Check sheet for the modelled part. Datum: model origin and axes. Units: mm. Face numbers are marked on the shaded views. A direction names the side the tool comes from. Round coordinates to 2 decimals unless told otherwise and drop trailing zeros. Write each loop counter-clockwise with the first axis right and the second up, starting at its lowest first coordinate (ties: lowest second). Pieces come first, ordered by that corner, then holes. Notation, with made-up numbers: (82, 42) -> (114, 42) arc R10 ccw to (114, 50) -> close; hole circle Ø1 at (59, -35.5). An arc over 180 degrees is marked (long way). One line per item, written item: value.
from build123d import *

# Parameters (mm, degrees)
SKIZZE1_W                       = 9.5
SKIZZE1_H                       = 11.093
SKIZZE1_W_2                     = 8.7
SKIZZE1_H_2                     = 4.7
SKIZZE1_H_3                     = 5.193
AUFSATZ_LINEAR_AUSTRAGEN1_DEPTH = 19.7
AUFSATZ_LINEAR_AUSTRAGEN2_DEPTH = 2.3
SCHNITT_LINEAR_AUSTRAGEN1_DEPTH = 13.7
SKIZZE4_W                       = 13.3
SKIZZE4_H                       = 5.193
SCHNITT_LINEAR_AUSTRAGEN2_DEPTH = 0.4
AUFSATZ_LINEAR_AUSTRAGEN3_DEPTH = 14.1
AUFSATZ_LINEAR_START            = -9.5
AUFSATZ_LINEAR_AUSTRAGEN4_DEPTH = 9.5
SCHNITT_LINEAR_AUSTRAGEN3_REACH = 39.021
SKIZZE7_W                       = 8.7
SKIZZE7_H                       = 0.4
SKIZZE8_W                       = 10
SKIZZE8_H                       = 5
AUFSATZ_LINEAR_AUSTRAGEN5_DEPTH = 0.4


with BuildPart() as part:
    # Skizze1 → Aufsatz-Linear austragen1 (new body)
    with BuildSketch(Plane(origin=(0, 0, 0), x_dir=(1, 0, 0), z_dir=(0, 1, 0))):
        with Locations((4.75, 5.5465)):
            Rectangle(SKIZZE1_W, SKIZZE1_H)
        with Locations((4.75, 2.75)):
            Rectangle(SKIZZE1_W_2, SKIZZE1_H_2, mode=Mode.SUBTRACT)
        with Locations((4.75, 8.0965)):
            Rectangle(SKIZZE1_W_2, SKIZZE1_H_3, mode=Mode.SUBTRACT)
    extrude(amount=AUFSATZ_LINEAR_AUSTRAGEN1_DEPTH)

    # Skizze2 → Aufsatz-Linear austragen2 (add)
    with BuildSketch(Plane.ZY):
        Polygon((-11.093, 0), (-8.093, 10.13), (-5.093, 0), align=None)
    aufsatz_linear_austragen2 = extrude(amount=AUFSATZ_LINEAR_AUSTRAGEN2_DEPTH)

    # Spiegeln1: Aufsatz-Linear austragen2 across plane
    add(aufsatz_linear_austragen2.mirror(Plane(origin=(4.75, 0, 0), x_dir=(0, 0, 1), z_dir=(1, 0, 0))))

    # Skizze3 → Schnitt-Linear austragen1 (cut)
    with BuildSketch(Plane.ZY.offset(2.3)):
        Polygon((-10.379677593, 1), (-5.806322407, 1), (-8.093, 8.721348004), align=None)
    extrude(amount=-SCHNITT_LINEAR_AUSTRAGEN1_DEPTH, mode=Mode.SUBTRACT)

    # Skizze4 → Schnitt-Linear austragen2 (cut)
    with BuildSketch(Plane.XZ):
        with Locations((4.75, -8.0965)):
            Rectangle(SKIZZE4_W, SKIZZE4_H)
    extrude(amount=-SCHNITT_LINEAR_AUSTRAGEN2_DEPTH, mode=Mode.SUBTRACT)

    # Skizze5 → Aufsatz-Linear austragen3 (add)
    with BuildSketch(Plane.ZY.offset(2.3)):
        Polygon((-20.977529946, -17.120508076), (-20.631119785, -17.320508076), (-10.631119785, 0), (-11.093, 0), align=None)
    extrude(amount=-AUFSATZ_LINEAR_AUSTRAGEN3_DEPTH)

    # Skizze6 → Aufsatz-Linear austragen4 (add)
    with BuildSketch(Plane.ZY.offset(AUFSATZ_LINEAR_START)):
        Polygon((-20.977529946, -17.120508076), (-11.093, 0), (-11.093, 14.7), align=None)
    extrude(amount=AUFSATZ_LINEAR_AUSTRAGEN4_DEPTH)

    # Skizze7 → Schnitt-Linear austragen3 (cut, up to next)
    with BuildSketch(Plane(origin=(0, 19.7, 0), x_dir=(1, 0, 0), z_dir=(0, 1, 0)), mode=Mode.PRIVATE) as schnitt_linear_austragen3_sk1:
        with Locations((4.75, 5.3)):
            Rectangle(SKIZZE7_W, SKIZZE7_H)
    schnitt_linear_austragen3_tool1 = extrude(schnitt_linear_austragen3_sk1.sketch, amount=-SCHNITT_LINEAR_AUSTRAGEN3_REACH, mode=Mode.PRIVATE) & part.part
    add(schnitt_linear_austragen3_tool1.solids().sort_by_distance((4.75, 19.7, -5.3))[0], mode=Mode.SUBTRACT)

    # Skizze8 → Aufsatz-Linear austragen5 (add)
    with BuildSketch(Plane(origin=(0, 4.603409902, -7.973339838), x_dir=(1, 0, 0), z_dir=(0, -0.5, 0.866025404))):
        with Locations((-7.3, -22.815559892)):
            Rectangle(SKIZZE8_W, SKIZZE8_H)
        with Locations((16.8, -22.815559892)):
            Rectangle(SKIZZE8_W, SKIZZE8_H)
    extrude(amount=-AUFSATZ_LINEAR_AUSTRAGEN5_DEPTH)


solid = part.part
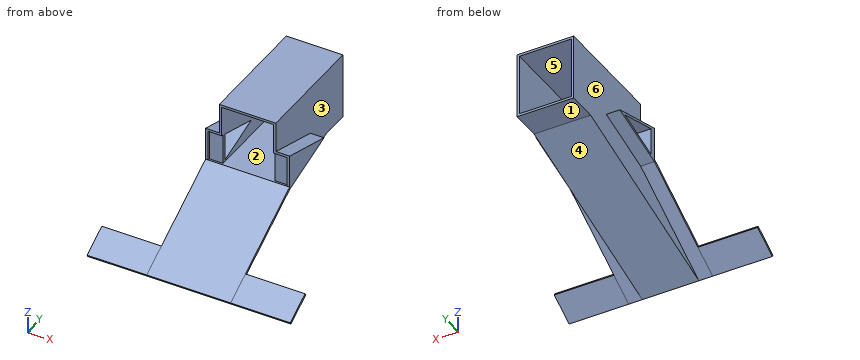
Item 1: Sectioned sample at D-D on y = -6. Enter the section's corners in (x, z).
Answer:
outline: (-2.3, -14.56) -> (0, -14.56) -> (0, -17.52) -> (9.5, -17.52) -> (9.5, -14.56) -> (11.8, -14.56) -> (11.8, -14.1) -> (-2.3, -14.1) -> close
Item 2: Sectioned sample at A-A on x = 3. Enter the section's corners in (y, z).
Answer:
outline: (-17.32, -20.63) -> (-17.12, -20.98) -> (14.7, -11.09) -> (19.7, -11.09) -> (19.7, -10.69) -> (0, -10.69) -> (0, -10.63) -> close; (0, -0.4) -> (19.7, -0.4) -> (19.7, 0) -> (0, 0) -> close
Item 3: Thickness scan on line 1 (X direction, y = 13, z = -3.25); line 2 (X direction, y = 5.5, z = -7.5); line 3 (Z direction, x = -1, y = 5). Record the ranges inside material, lowest first.
Answer:
line 1: x = 0 to 0.4, 9.1 to 9.5
line 2: x = 11.4 to 11.8
line 3: z = -9.61 to -9.2, -6.99 to -6.57
Item 4: Sectioned sample at B-B on z = -3.25. Enter the section's corners in (x, y).
Answer:
outline: (0, 0) -> (0.4, 0) -> (0.4, 19.7) -> (0, 19.7) -> close; (9.1, 0) -> (9.5, 0) -> (9.5, 19.7) -> (9.1, 19.7) -> close
Item 5: Depth check by flat-ended pin: P1, Ø2, axis at y = -10, z = -16, coming from the +X side; P2, Ø3, axis at y = 6, z = -5.5, coming from the -X side; P3, Ø0.7, axis at x = -1.5, z = -7.5, coming from the -Y side; P4, Ø12, axis at y = -8, z = -5.5, coming from the -X side. Enter the tip coordinate at first touch or a pass-through.
Answer:
P1: stops at x = 11.8
P2: stops at x = -2.3
P3: stops at y = 0.4
P4: passes through
Item 6: Tool access check on the marked faces 4, 5 and 6. Record the directions out of +Z, -Z, +X, -X, +Y, -Y that give a thin tool (end or side, any length) a straight path to the whole face; none if there is none.
Answer:
face 4: -Z, +X, -X, +Y
face 5: +Y, -Y
face 6: -X, +Y
Item 7: Mould release check, pull along X, two halves, no side actions. Record for the marked faces 1, 2 and 3: pulls with the +X half, pulls with the -X half, needs draft (parallel to the pull), parting line crosses it, or undercut.
Answer:
face 1: needs draft
face 2: undercut
face 3: pulls with the +X half
Item 8: Sectioned sample at C-C on z = -9. Enter the section's corners in (x, y).
Answer:
outline: (-2.3, 0) -> (-1.9, 0) -> (-1.9, 0.4) -> (0.4, 0.4) -> (0.4, 1) -> (-2.3, 1) -> close; (-2.3, 5.66) -> (0.4, 5.66) -> (0.4, 19.7) -> (0, 19.7) -> (0, 7.07) -> (-2.3, 7.07) -> close; (9.1, 0.4) -> (11.4, 0.4) -> (11.4, 0) -> (11.8, 0) -> (11.8, 7.07) -> (9.5, 7.07) -> (9.5, 19.7) -> (9.1, 19.7) -> (9.1, 5.66) -> (11.4, 5.66) -> (11.4, 1) -> (9.1, 1) -> close
